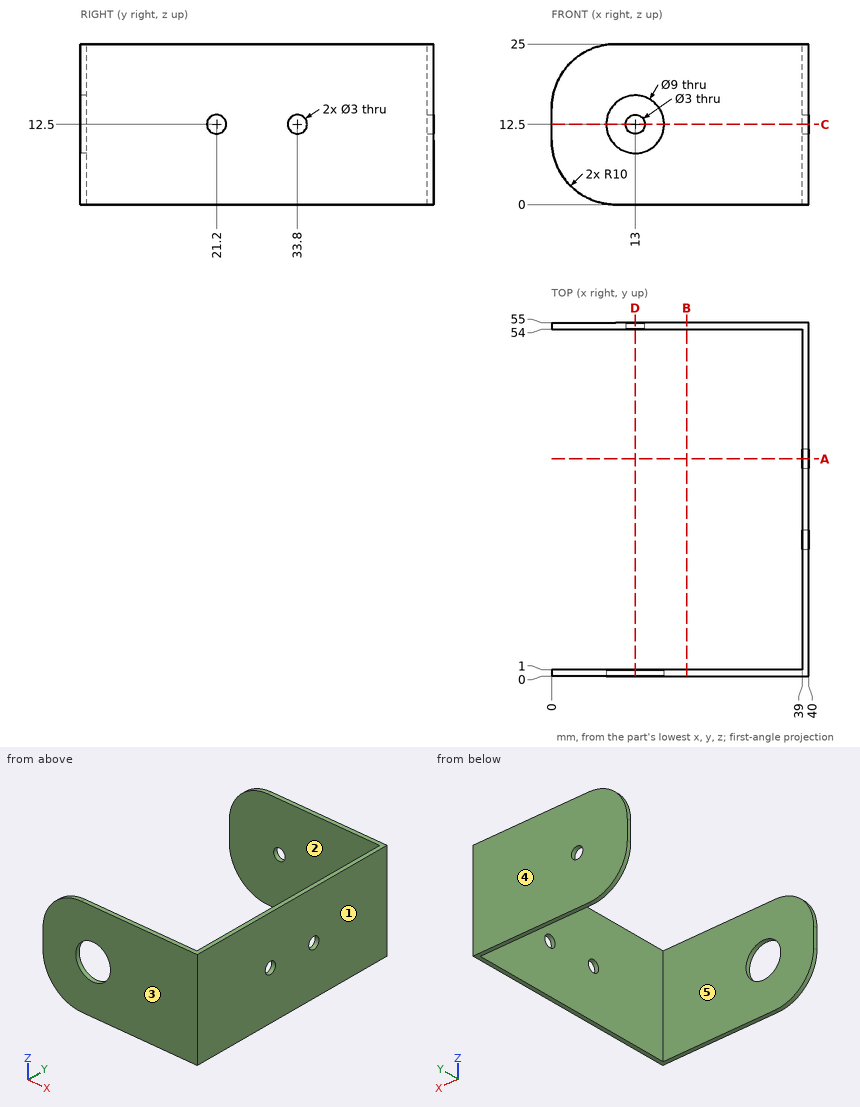
Geometry check sheet. Reference: drawing and pictorial views, mm from the part's lowest x, y, z. A direction names the side the tool comes from. Coordinates: 2 decimals unless noted, no trailing zeros. Loops run counter-clockwise (first coordinate to the right, second up) from the corner with the lowest first, then second, coordinate; pieces in that order, holes last.
1) Sectioned sample at A-A (y = 33.8). Record the boundary of the cut face in (x, z).
2) Gauge pin test, flat ends, axial feed: pin 1 (4 mm diameter, centred on x = 13, z = 12.5, fed in from -Y); pin 2 (7.5 mm diameter, centred on y = 31.5, z = 7, fed in from -X). Record the tip position at first contact, or that the pin passes through.
3) Sectioned sample at D-D (x = 13). Record the boundary of the cut face in (y, z).
4) Access from +Z, -Z, +X, -X, +Y, -Y to the whole of each face (thin tool, end or side, straight path). Record for the marked faces 1 and 2.
5) Material ranges on probe 1 along Y at (x, z) = (28.5, 20.25); probe 2 along X at (y, z) = (40.5, 9.5); probe 3 along Y at (x, z) = (14, 15.75), recorded low to high.
6) Sectioned sample at B-B (x = 21). Record the boundary of the cut face in (y, z), and give its area (3 significant figures).
7) Sectioned sample at C-C (z = 12.5). Record the boundary of the cut face in (x, y), and give its area (3 significant figures).
8) Release check for a two-part mould opening along Y. For the marked faces 3, 4 and 5 record: released by +Y, released by -Y, zero draft, split by the parting line, or undercut.
Check sheet entries:
1. outline: (39, 0) - (40, 0) - (40, 11) - (39, 11) - close; (39, 14) - (40, 14) - (40, 25) - (39, 25) - close
2. pin 1: stops at y = 54
2. pin 2: stops at x = 39
3. outline: (0, 0) - (1, 0) - (1, 8) - (0, 8) - close; (0, 17) - (1, 17) - (1, 25) - (0, 25) - close; (54, 0) - (55, 0) - (55, 11) - (54, 11) - close; (54, 14) - (55, 14) - (55, 25) - (54, 25) - close
4. face 1: +Z, -Z, +X, +Y, -Y
4. face 2: +Z, -Z, -X
5. probe 1: y = 0 to 1, 54 to 55
5. probe 2: x = 39 to 40
5. probe 3: y = 54 to 55
6. outline: (0, 0) - (1, 0) - (1, 25) - (0, 25) - close; (54, 0) - (55, 0) - (55, 25) - (54, 25) - close
6. area: 50.0 mm2
7. outline: (0, 0) - (8.5, 0) - (8.5, 1) - (0, 1) - close; (0, 54) - (11.5, 54) - (11.5, 55) - (0, 55) - close; (14.5, 54) - (39, 54) - (39, 35.3) - (40, 35.3) - (40, 55) - (14.5, 55) - close; (17.5, 0) - (40, 0) - (40, 19.7) - (39, 19.7) - (39, 1) - (17.5, 1) - close; (39, 22.7) - (40, 22.7) - (40, 32.3) - (39, 32.3) - close
7. area: 115 mm2
8. face 3: released by -Y
8. face 4: released by +Y
8. face 5: undercut
